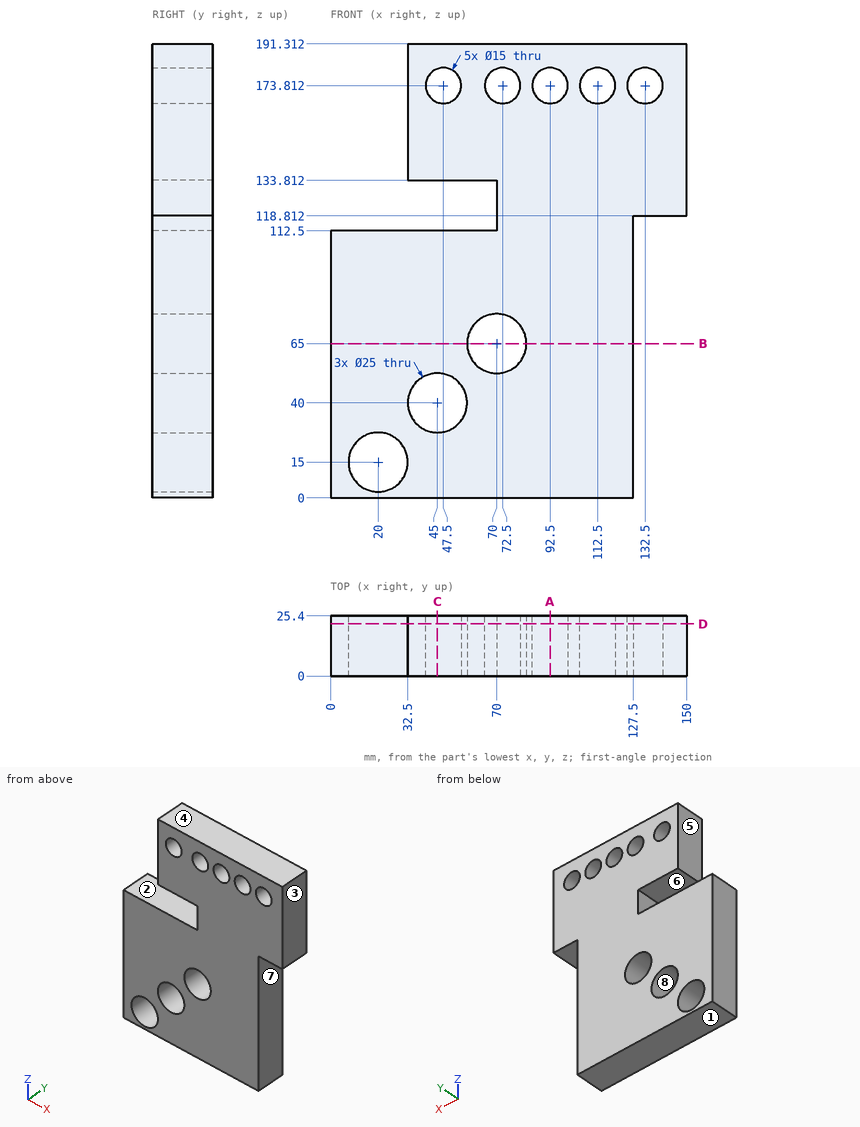
Input: dimensioned drawing with shaded views. Units: mm. Origin: part minimum x, y, z. A direction names the side the tool comes from. Round coordinates to 2 decimals unless told otherwise and drop trailing zeros. Loops run counter-clockwise (first coordinate to the right, second up) from the corner with the lowest first, then second, coordinate; pieces in that order, holes last. Notation, with made-up numbers: (37.25, -10.75) -> (87.25, -10.75) arc R16 cw to (87.25, 18.25) -> close; hole circle Ø11 at (44.25, 79.25). An arc over 180 degrees is marked (long way). Answer as a JSON object with one key per item and string values. Group by question number.
Q1. Access query for the marked faces 5, 6, 7 and 8. Directions: +Z, -Z, +X, -X, +Y, -Y. A direction counts if a zero-diameter tool reaches every point of the face in a straight line with its end or side. Return the directions, or none.
Q2. Section query A-A (x = 92.5). Output: boundary loops of the cut face in (y, z).
Q3. Contact query for a flat-ended pin moving along its axis: P1, Ø1, axis at y = 17.5, z = 49.5, coming from the +X side. Output: stop coordinate, or through.
Q4. Section query B-B (z = 65). Output: boundary loops of the cut face in (x, y), plus the area to 3 significant figures.
Q5. Section query D-D (y = 22). State how many separate pieces and enclosed holes the cut face has, plus the area to 3 significant figures.
Q6. Ray query, line 1 (Z direction, x = 47.5, y = 18.25); line 2 (Z direction, x = 132.5, y = 10.5); line 3 (Z direction, x = 45, y = 14.5). Return the intervals inside material, ascending. Write a range as from..to.
Q7. Section query C-C (x = 45). Output: boundary loops of the cut face in (y, z), plus the area to 3 significant figures.
Q8. Mould query, pull axis Z, two halves, no side actions, for the marked faces 1, 2, 3 and 4. Classes: pulls with the +Z half, pulls with the -Z half, needs draft (parallel to the pull), parting line crosses it, or undercut.
Completed:
{
 "1": {"face 5": "+Z, -X, +Y, -Y", "face 6": "-X, +Y, -Y", "face 7": "-Z, +X, +Y, -Y", "face 8": "+Y, -Y"},
 "2": {"outline": "(0, 0) -> (25.4, 0) -> (25.4, 166.31) -> (0, 166.31) -> close; (0, 181.31) -> (25.4, 181.31) -> (25.4, 191.31) -> (0, 191.31) -> close"},
 "3": {"P1": "x = 127.5"},
 "4": {"outline": "(0, 0) -> (57.5, 0) -> (57.5, 25.4) -> (0, 25.4) -> close; (82.5, 0) -> (127.5, 0) -> (127.5, 25.4) -> (82.5, 25.4) -> close", "area": "2,600 mm²"},
 "5": {"separate pieces": "1", "enclosed holes": "8", "area": "20,300 mm²"},
 "6": {"line 1": "0..27.75, 52.25..112.5, 133.81..166.31, 181.31..191.31", "line 2": "118.81..166.31, 181.31..191.31", "line 3": "0..27.5, 52.5..112.5, 133.81..166.74, 180.88..191.31"},
 "7": {"outline": "(0, 0) -> (25.4, 0) -> (25.4, 27.5) -> (0, 27.5) -> close; (0, 52.5) -> (25.4, 52.5) -> (25.4, 112.5) -> (0, 112.5) -> close; (0, 133.81) -> (25.4, 133.81) -> (25.4, 166.74) -> (0, 166.74) -> close; (0, 180.88) -> (25.4, 180.88) -> (25.4, 191.31) -> (0, 191.31) -> close", "area": "3,320 mm²"},
 "8": {"face 1": "pulls with the -Z half", "face 2": "undercut", "face 3": "needs draft", "face 4": "pulls with the +Z half"}
}
